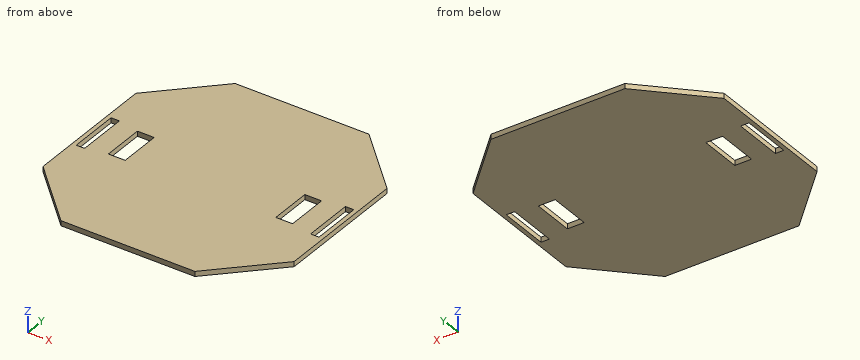
from build123d import *

# Parameters (mm, degrees)
F1_DEPTH = 6


with BuildPart() as f1:
    # F0 (on Top) → F1 (new body)
    with BuildSketch(Plane.XY):
        Polygon((80, 150), (0, 150), (0, 0), (90, 0), (90, 25), (110, 25), (110, 0), (135, 0), (135, 30), (145, 30), (145, 0), (150, 0), (150, 80), align=None)
        Polygon((0, 150), (-80, 150), (-150, 80), (-150, 0), (-145, 0), (-145, 30), (-135, 30), (-135, 0), (-110, 0), (-110, 25), (-90, 25), (-90, 0), (0, 0), align=None)
        Polygon((-145, 0), (-150, 0), (-150, -80), (-80, -150), (0, -150), (0, 0), (-90, 0), (-90, -25), (-110, -25), (-110, 0), (-135, 0), (-135, -30), (-145, -30), align=None)
        Polygon((90, 0), (0, 0), (0, -150), (80, -150), (150, -80), (150, 0), (145, 0), (145, -30), (135, -30), (135, 0), (110, 0), (110, -25), (90, -25), align=None)
    extrude(amount=F1_DEPTH)


solid = f1.part
Geometry check sheet. Reference: the model listing, model coordinates, mm. Round coordinates to 2 decimals unless told otherwise and drop trailing zeros. Loops run counter-clockwise (first coordinate to the right, second up) from the corner with the lowest first, then second, coordinate; pieces in that order, holes last.
Item 1: Thickness scan on line 1 (X direction, y = -18.5, z = 4.65); line 2 (X direction, y = 95, z = 1.8); line 3 (Y direction, x = -130.5, z = 0.75). Record the ranges inside material, lowest first.
Item 2: Cross-section at B-B on z = 1.75. Record the boundary of the cut face in (x, y).
Item 3: Cross-section at D-D on y = -116.5. Record the boundary of the cut face in (x, z).
Item 4: Cross-section at C-C on x = 106. Record the boundary of the cut face in (y, z), then the cut area to 3 significant figures.
Item 5: Cross-section at A-A on x = -103. Record the boundary of the cut face in (y, z).
Item 6: Gauge pin test, flat ends, axial feed: pin 1 (1.8 mm diameter, centred on x = 138.5, z = 2, fed in from -Y); pin 2 (1.8 mm diameter, centred on x = 141, z = 4, fed in from +Y); pin 3 (1 mm diameter, centred on y = -83.5, z = 4.5, fed in from +X); pin 4 (4 mm diameter, centred on x = -83, y = -25, fed in from -Z). Record the tip position at first contact, or that the pin passes through.
Answer sheet:
1. line 1: x = -150 to -145, -135 to -110, -90 to 90, 110 to 135, 145 to 150
1. line 2: x = -135 to 135
1. line 3: y = -99.5 to 99.5
2. outline: (-150, -80) - (-80, -150) - (80, -150) - (150, -80) - (150, 80) - (80, 150) - (-80, 150) - (-150, 80) - close; hole (-145, -30) - (-135, -30) - (-135, 30) - (-145, 30) - close; hole (-110, -25) - (-90, -25) - (-90, 25) - (-110, 25) - close; hole (90, -25) - (110, -25) - (110, 25) - (90, 25) - close; hole (135, -30) - (145, -30) - (145, 30) - (135, 30) - close
3. outline: (-113.5, 0) - (113.5, 0) - (113.5, 6) - (-113.5, 6) - close
4. outline: (-124, 0) - (-25, 0) - (-25, 6) - (-124, 6) - close; (25, 0) - (124, 0) - (124, 6) - (25, 6) - close
4. area: 1,190 mm2
5. outline: (-127, 0) - (-25, 0) - (-25, 6) - (-127, 6) - close; (25, 0) - (127, 0) - (127, 6) - (25, 6) - close
6. pin 1: stops at y = -92.4
6. pin 2: stops at y = 89.9
6. pin 3: stops at x = 147
6. pin 4: stops at z = 0
